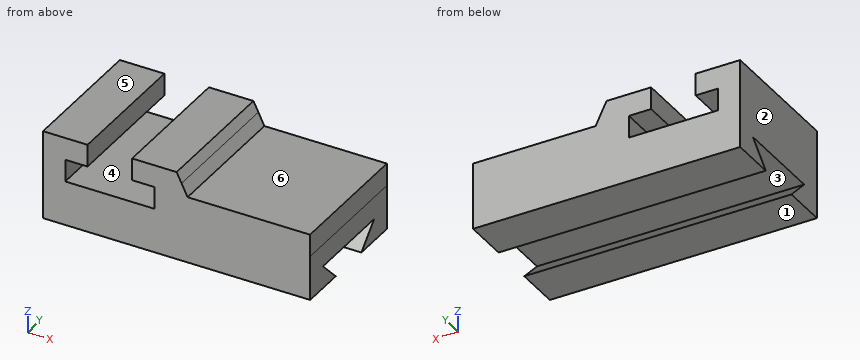
```python
from build123d import *

# Parameters (mm, degrees)
F1_DEPTH = 76.2
F3_DEPTH = 152.4


# Not quite as in the source:
# - a feature names something its author has since deleted; it is built from what else it names


with BuildPart() as f1:
    # F0 (on Front) → F1 (new body)
    with BuildSketch(Plane.XZ):
        Polygon((-76.2, 25.4), (-76.2, 0), (76.2, 0), (76.2, 25.4), (76.1036425829, 38.1), (6.2536425829, 38.1), (2.8439569287, 45.1241247356), (0, 50.8), (-25.4, 50.8), (-25.4, 38.1), (-12.7, 38.1), (-12.7, 25.4), (-63.5, 25.4), (-63.5, 38.1), (-50.8, 38.1), (-50.8, 50.8), (-76.2, 50.8), align=None)
    extrude(amount=F1_DEPTH)

    # F2 (on face) → F3 (cut)
    with BuildSketch(Plane.YZ.offset(76.2)):
        Polygon((-63.5, 12.7), (-50.8, 0), (-38.1, 0), (-38.1, 12.7), align=None)
        Polygon((-38.1, 12.7), (-38.1, 0), (-25.4, 0), (-12.7, 12.7), align=None)
    extrude(amount=-F3_DEPTH, mode=Mode.SUBTRACT)


solid = f1.part
```
The model under review builds one solid part; all positions refer to its coordinate system, in mm. Face numbers are marked on the shaded views. A direction names the side the tool comes from. Round coordinates to 2 decimals unless told otherwise and drop trailing zeros. Write each loop counter-clockwise with the first axis right and the second up, starting at its lowest first coordinate (ties: lowest second). Pieces come first, ordered by that corner, then holes.
(1) Wall thickness on L1, parallel to Z at x = -57.5, y = -38; L2, parallel to X at y = -18.5, z = 29.5; L3, parallel to X at y = -3, z = 33.5: over which ranges is each line inside the solid? List them lowest first.
(2) We need section B-B on z = 11. Give the boundary of the cut face in (x, y), and give its area (3 significant figures).
(3) We need section C-C on y = -60. Give the boundary of the cut face in (x, z), and give its area (3 significant figures).
(4) Mouldability with a two-part tool opening along Z and no side actions: class the marked faces 1, 2 and 3 as +Z half, -Z half, draft (parallel to the pull), parting line (faces both ways), or undercut.
(5) Machinability: for the marked faces 4, 5 and 6, which of the approach directions +Z, -Z, +X, -X, +Y, -Y give a long, thin tool a straight path to every point of the face, cutting with its end or side? Answer none if there is none.
(6) We need section A-A on x = -60. Give the boundary of the cut face in (y, z), and give its area (3 significant figures).
(7) We need section D-D on x = -30.5. Give the boundary of the cut face in (y, z), and give its area (3 significant figures).
(8) Insertion check: pin 1 (10 mm diameter, centred on y = -36.5, z = 33, fed in from +X); pin 2 (1 mm diameter, centred on x = 36, y = -27.5, fed in from -Z); pin 3 (1 mm diameter, centred on x = 18.5, y = -59, fed in from +Z). Each pin has a flat end and moves straight along its axis. Give the tip position at first contact, or say it passes through.
Findings below:
1. L1: z = 12.7 to 25.4, 38.1 to 50.8
1. L2: x = -76.2 to -63.5, -12.7 to 76.17
1. L3: x = -76.2 to -63.5, -12.7 to 76.14
2. outline: (-76.2, -76.2) - (76.2, -76.2) - (76.2, -61.8) - (-76.2, -61.8) - close; (-76.2, -14.4) - (76.2, -14.4) - (76.2, 0) - (-76.2, 0) - close
2. area: 4,390 mm2
3. outline: (-76.2, 0) - (76.2, 0) - (76.2, 9.2) - (-76.2, 9.2) - close; (-76.2, 12.7) - (76.2, 12.7) - (76.2, 25.4) - (76.1, 38.1) - (6.25, 38.1) - (2.84, 45.12) - (0, 50.8) - (-25.4, 50.8) - (-25.4, 38.1) - (-12.7, 38.1) - (-12.7, 25.4) - (-63.5, 25.4) - (-63.5, 38.1) - (-50.8, 38.1) - (-50.8, 50.8) - (-76.2, 50.8) - close
3. area: 5,310 mm2
4. face 1: -Z half
4. face 2: draft
4. face 3: undercut
5. face 4: +Y, -Y
5. face 5: +Z, +X, -X, +Y, -Y
5. face 6: +Z, +X, +Y, -Y
6. outline: (-76.2, 0) - (-50.8, 0) - (-63.5, 12.7) - (-12.7, 12.7) - (-25.4, 0) - (0, 0) - (0, 25.4) - (-76.2, 25.4) - close; (-76.2, 38.1) - (0, 38.1) - (0, 50.8) - (-76.2, 50.8) - close
6. area: 2,420 mm2
7. outline: (-76.2, 0) - (-50.8, 0) - (-63.5, 12.7) - (-12.7, 12.7) - (-25.4, 0) - (0, 0) - (0, 25.4) - (-76.2, 25.4) - close
7. area: 1,450 mm2
8. pin 1: stops at x = 76.18
8. pin 2: stops at z = 12.7
8. pin 3: stops at z = 38.1
